Read the model definition and answer for the solid it produces. Units are mm, in the model's axes. Face numbers are marked on the shaded views. A direction names the side the tool comes from. Coordinates: 2 decimals unless noted, no trailing zeros. Write each loop counter-clockwise with the first axis right and the second up, starting at its lowest first coordinate (ties: lowest second). Pieces come first, ordered by that corner, then holes. Notation, with made-up numbers: (30.25, 63.5) -> (46.25, 63.5) arc R31 ccw to (46.25, 95.5) -> close; hole circle Ø9 at (88, 45). An arc over 180 degrees is marked (long way). Return JSON: item names as keys, results as strings.
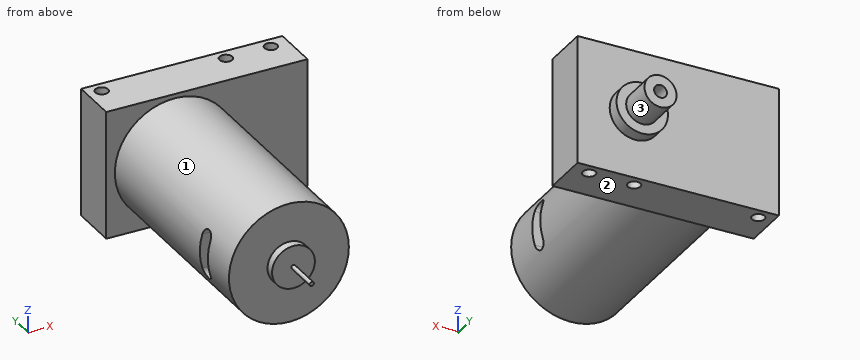
from build123d import *

# Parameters (mm, degrees)
SKETCH_1_W          = 47
SKETCH_1_H          = 30
EXTRUDE_1_DEPTH     = 11
SKETCH_2_R          = 6
EXTRUDE_2_DEPTH     = 3
SKETCH_3_R          = 3.75277675
EXTRUDE_3_DEPTH     = 8
SKETCH_4_R          = 14
EXTRUDE_4_DEPTH     = 50
SKETCH_5_R          = 5
EXTRUDE_5_DEPTH     = 2
SKETCH_6_R          = 1.5
CUT_EXTRUDE_1_DEPTH = 31
CUT_EXTRUDE_2_DEPTH = 48
SKETCH_9_R          = 1.5
CUT_EXTRUDE_3_DEPTH = 8
SKETCH_11_R         = 0.5
EXTRUDE_6_DEPTH     = 8


with BuildPart() as part:
    # 草图1 → 凸台-拉伸1 (new body)
    with BuildSketch(Plane(origin=(0, 0, 0), x_dir=(1, 0, 0), z_dir=(0, 1, 0))):
        with Locations((23.5, -15)):
            Rectangle(SKETCH_1_W, SKETCH_1_H)
    extrude(amount=EXTRUDE_1_DEPTH)

    # 草图2 → 凸台-拉伸2 (add)
    with BuildSketch(Plane(origin=(0, 11, 0), x_dir=(1, 0, 0), z_dir=(0, 1, 0))):
        with Locations((33.5, -15)):
            Circle(SKETCH_2_R)
    extrude(amount=EXTRUDE_2_DEPTH)

    # 草图3 → 凸台-拉伸3 (add)
    with BuildSketch(Plane(origin=(0, 14, 0), x_dir=(1, 0, 0), z_dir=(0, 1, 0))):
        with Locations((33.5, -15)):
            Circle(SKETCH_3_R)
    extrude(amount=EXTRUDE_3_DEPTH)

    # 草图4 → 凸台-拉伸4 (add)
    with BuildSketch(Plane.XZ):
        with Locations((16, 15)):
            Circle(SKETCH_4_R)
    extrude(amount=EXTRUDE_4_DEPTH)

    # 草图5 → 凸台-拉伸5 (add)
    with BuildSketch(Plane.XZ.offset(50)):
        with Locations((16, 15)):
            Circle(SKETCH_5_R)
    extrude(amount=EXTRUDE_5_DEPTH)

    # 草图6 → 切除-拉伸1 (cut, through all)
    with BuildSketch(Plane.XY.offset(30)):
        with Locations((3.340757383, 8.25)):
            Circle(SKETCH_6_R)
        with Locations((32.340757383, 8.25)):
            Circle(SKETCH_6_R)
        with Locations((42.840757383, 8.25)):
            Circle(SKETCH_6_R)
    extrude(amount=-CUT_EXTRUDE_1_DEPTH, mode=Mode.SUBTRACT)

    # 草图7 → 切除-拉伸2 (cut, through all)
    with BuildSketch(Plane.ZY):
        with BuildLine():
            Line((11, -37.25), (19, -37.25))
            ThreePointArc((19, -37.25), (20.75, -39), (19, -40.75))
            Line((19, -40.75), (11, -40.75))
            ThreePointArc((11, -40.75), (9.25, -39), (11, -37.25))
        make_face()
    extrude(amount=-CUT_EXTRUDE_2_DEPTH, mode=Mode.SUBTRACT)

    # 草图9 → 切除-拉伸3 (cut)
    with BuildSketch(Plane(origin=(0, 22, 0), x_dir=(1, 0, 0), z_dir=(0, 1, 0))):
        with Locations((33.5, -15)):
            Circle(SKETCH_9_R)
    extrude(amount=-CUT_EXTRUDE_3_DEPTH, mode=Mode.SUBTRACT)

    # 草图11 → 凸台-拉伸6 (add)
    with BuildSketch(Plane.XZ.offset(52)):
        with Locations((16, 15)):
            Circle(SKETCH_11_R)
    extrude(amount=EXTRUDE_6_DEPTH)


solid = part.part
1. A tool of negligible diameter and unlimited length cuts with its end or side. For the marked faces 1, 2 and 3, from which of +Z, -Z, +X, -X, +Y, -Y can it reach the whole face along a straight path? Write none if from no direction.
Taken from the geometry:
{"face 1": "-Y", "face 2": "-Z, +X, -X, +Y, -Y", "face 3": "+Y"}
2. The part is cut by section D-D (x = 22.5). Determine the outline of the cut face in (y, z).
Taken from the geometry:
{"outline": "(-50, 2.6) -> (0, 2.6) -> (0, 0) -> (11, 0) -> (11, 30) -> (0, 30) -> (0, 27.4) -> (-50, 27.4) -> close; hole (-40.75, 11) arc R1.75 ccw to (-37.25, 11) -> (-37.25, 19) arc R1.75 ccw to (-40.75, 19) -> close"}
3. The part is cut by section C-C (x = 33). Determine the outline of the cut face in (y, z).
Taken from the geometry:
{"outline": "(0, 0) -> (6.9, 0) -> (6.9, 30) -> (0, 30) -> close; (9.6, 0) -> (11, 0) -> (11, 9.02) -> (14, 9.02) -> (14, 11.28) -> (22, 11.28) -> (22, 13.59) -> (14, 13.59) -> (14, 16.41) -> (22, 16.41) -> (22, 18.72) -> (14, 18.72) -> (14, 20.98) -> (11, 20.98) -> (11, 30) -> (9.6, 30) -> close"}
4. Consider L1, parallel to X at y = 7.5, z = 28.75; L2, parallel to Y at x = 14, z = 14; L3, parallel to Y at x = 26, z = 3.5. Determine where each line is inside the solid, lowest interval first.
Taken from the geometry:
{"L1": "x = 0 to 2.04, 4.64 to 31.04, 33.64 to 41.54, 44.14 to 47", "L2": "y = -52 to -40.75, -37.25 to 11", "L3": "y = 0 to 11"}
5. The part is cut by section A-A (y = 8.25). Determine the outline of the cut face in (x, z), then the cut area to 3 significant figures.
Taken from the geometry:
{"outline": "(0, 0) -> (1.84, 0) -> (1.84, 30) -> (0, 30) -> close; (4.84, 0) -> (30.84, 0) -> (30.84, 30) -> (4.84, 30) -> close; (33.84, 0) -> (41.34, 0) -> (41.34, 30) -> (33.84, 30) -> close; (44.34, 0) -> (47, 0) -> (47, 30) -> (44.34, 30) -> close", "area": "1,140 mm2"}
6. The part is cut by section B-B (z = 3.75). Determine the outline of the cut face in (x, y).
Taken from the geometry:
{"outline": "(0, 0) -> (7.67, 0) -> (7.67, -50) -> (24.33, -50) -> (24.33, 0) -> (47, 0) -> (47, 11) -> (0, 11) -> close; hole circle Ø3 at (3.34, 8.25); hole circle Ø3 at (32.34, 8.25); hole circle Ø3 at (42.84, 8.25)"}
7. Flat-ended cylindrical pins translate along their axes: pin 1 Ø12 at (x, y) = (13.5, -14) entering from +Z; pin 2 Ø2.5 at (x, z) = (33.5, 15) entering from +Y; pin 3 Ø1 at (x, z) = (22.5, 10) entering from +Y; pin 4 Ø6 at (y, z) = (12, 11) entering from -X. Find the tip coordinate at first contact, or state that the pin passes through.
Taken from the geometry:
{"pin 1": "stops at z = 29", "pin 2": "stops at y = 14", "pin 3": "stops at y = 11", "pin 4": "stops at x = 0"}
